from build123d import *

# Parameters (mm, degrees)
SKETCH1_W                                           = 115
SKETCH1_H                                           = 35
BOSS_EXTRUDE1_DEPTH                                 = 5
CSK_FOR_M3_FLAT_COUNTERSUNK_HEAD_SCREW1_D           = 3.4
CSK_FOR_M3_FLAT_COUNTERSUNK_HEAD_SCREW1_CSINK_D     = 6.3
CSK_FOR_M3_FLAT_COUNTERSUNK_HEAD_SCREW1_CSINK_ANGLE = 90


with BuildPart() as part:
    # Sketch1 → Boss-Extrude1 (new body)
    with BuildSketch(Plane(origin=(0, 0, 0), x_dir=(1, 0, 0), z_dir=(0, 1, 0))):
        with Locations((57.5, 17.5)):
            Rectangle(SKETCH1_W, SKETCH1_H)
    extrude(amount=-BOSS_EXTRUDE1_DEPTH)

    # CSK for M3 Flat Countersunk Head Screw1 (through all)
    with Locations(Plane(origin=(0, 0, 0), x_dir=(1, 0, 0), z_dir=(0, 1, 0))):
        with Locations((2.5, 25), (2.5, 10), (112.5, 25), (112.5, 10)):
            CounterSinkHole(CSK_FOR_M3_FLAT_COUNTERSUNK_HEAD_SCREW1_D / 2, CSK_FOR_M3_FLAT_COUNTERSUNK_HEAD_SCREW1_CSINK_D / 2, counter_sink_angle=CSK_FOR_M3_FLAT_COUNTERSUNK_HEAD_SCREW1_CSINK_ANGLE)


solid = part.part
Check sheet for the modelled part. Datum: model origin and axes. Units: mm. Round coordinates to 2 decimals unless told otherwise and drop trailing zeros. Order: outer loops, then holes, each group sorted by start corner. A loop starts at its lowest first (then second) coordinate and runs counter-clockwise, first axis right, second up.
(1) Cross-section at B-B, the plane z = -25. Enter the section's corners in (x, y), and give its area (3 significant figures).
(2) Scan lines: probe 1 along X at (y, z) = (-2.2, -10); probe 2 along Z at (x, y) = (2.5, -3.95); probe 3 along X at (y, z) = (-2.7, -24). Record each from-to range of solid material in increasing order.
(3) Go/stop test with flat-tipped pins: P1, Ø2, axis at y = -3, z = -15, coming from the -X side; P2, Ø2, axis at x = 2.5, z = -10, coming from the +Y side; P3, Ø4, axis at x = 112.5, z = -10, coming from the +Y side. Record where each tip stops, or that it passes through.
(4) Cross-section at A-A, the plane x = 2.5. Enter the section's corners in (y, z).
(5) Draft check along X on faces 1 (the flat face through (57, -2, -35)), 2 (the flat face through (0, -2, -17)), 3 (the conical face through (110.66, -1.22, -25.58)), 4 (the cylindrical face through (114.2, -3.25, -25.07)). Enter one of: pulls with the +X half, pulls with the -X half, needs draft (parallel to the pull), parting line crosses it, or undercut.
Check sheet entries:
1. outline: (0, -5) - (0.8, -5) - (0.8, -1.45) - (0, -0.65) - close; (4.2, -5) - (110.8, -5) - (110.8, -1.45) - (109.35, 0) - (5.65, 0) - (4.2, -1.45) - close; (114.2, -5) - (115, -5) - (115, -0.65) - (114.2, -1.45) - close
1. area: 537 mm2
2. probe 1: x = 0 to 0.8, 4.2 to 110.8, 114.2 to 115
2. probe 2: z = -35 to -26.7, -23.3 to -11.7, -8.3 to 0
2. probe 3: x = 0 to 1.13, 3.87 to 111.13, 113.87 to 115
3. P1: stops at x = 0
3. P2: passes through
3. P3: stops at y = -1.15
4. outline: (-5, -35) - (0, -35) - (0, -28.15) - (-1.45, -26.7) - (-5, -26.7) - close; (-5, -23.3) - (-1.45, -23.3) - (0, -21.85) - (0, -13.15) - (-1.45, -11.7) - (-5, -11.7) - close; (-5, -8.3) - (-1.45, -8.3) - (0, -6.85) - (0, 0) - (-5, 0) - close
5. face 1: needs draft
5. face 2: pulls with the -X half
5. face 3: undercut
5. face 4: undercut
